The listing builds one solid part. Answer for the finished solid, in the listing's coordinates (mm). A direction names the side the tool comes from. Coordinates: 2 decimals unless noted, no trailing zeros. Write each loop counter-clockwise with the first axis right and the second up, starting at its lowest first coordinate (ties: lowest second). Pieces come first, ordered by that corner, then holes. Notation, with made-up numbers: M 69,-13 L 112,-13 A26 cw 112,16 Z; hole C -23.5,25 d3. An arc over 180 degrees is marked long. Answer as a JSON object with one key per item and string values. Group by question number.
from build123d import *

# Parameters (mm, degrees)
SKETCH1_R           = 6
SKETCH1_R_2         = 2.5
BOSS_EXTRUDE1_DEPTH = 11.75
SKETCH2_R           = 2.413
SKETCH3_R           = 1.5
CUT_EXTRUDE1_DEPTH  = 12
CHAMFER1_SIZE       = 0.508
CHAMFER2_SIZE       = 0.254


with BuildPart() as part:
    # Sketch1 → Boss-Extrude1 (new body)
    with BuildSketch(Plane(origin=(0, 0, 0), x_dir=(0, 0, -1), z_dir=(1, 0, 0))):
        Circle(SKETCH1_R)
        Circle(SKETCH1_R_2, mode=Mode.SUBTRACT)
    extrude(amount=-BOSS_EXTRUDE1_DEPTH)

    # Sketch2 → Cut-Revolve1 (revolve, cut)
    with BuildSketch(Plane(origin=(0, 0, 0), x_dir=(1, 0, 0), z_dir=(0, 1, 0))):
        with Locations((-3.629714112, 7.913)):
            Circle(SKETCH2_R)
    revolve(axis=Axis((0, 0, 0), (1, 0, 0)), mode=Mode.SUBTRACT)

    # Sketch3 → Cut-Extrude1 (cut)
    with BuildSketch(Plane(origin=(0, 0, 0), x_dir=(1, 0, 0), z_dir=(0, 1, 0))):
        with Locations((-8, 0)):
            Circle(SKETCH3_R)
    extrude(amount=CUT_EXTRUDE1_DEPTH, mode=Mode.SUBTRACT)

    # Chamfer1
    chamfer1_edges = [part.edges().sort_by_distance(p)[0] for p in [
        (0, 0, 6),
        (-11.75, 0, 6),
    ]]
    chamfer(chamfer1_edges, length=CHAMFER1_SIZE)

    # Chamfer2
    chamfer2_edges = [part.edges().sort_by_distance(p)[0] for p in [
        (0, 0, 2.5),
    ]]
    chamfer(chamfer2_edges, length=CHAMFER2_SIZE)


solid = part.part
Item 1: Consider L1, parallel to X at y = 3.15, z = 0; L2, parallel to Z at x = -8, y = 4.55; L3, parallel to Y at x = -6.75, z = 0. Determine where each line is inside the solid, lowest interval first. Write a range as from..to.
Item 2: A cutting plane is placed at B-B, the plane z = 0. Write down the section's boundary in (x, y), and give its area (3 significant figures).
Item 3: A tool of negligible diameter and unlimited length cuts with its end or side. For faces 1 (the face through (-11.75, 3, 0)), 2 (the face through (-6.614, 3.974, 0.575)), from which of +Z, -Z, +X, -X, +Y, -Y can it reach the whole face along a straight path? Write none if from no direction.
Item 4: For a pull along Z with two mould halves and no side action, classify faces 3 (the face through (-8.128, -5.857, 1.301)), 4 (the face through (0, 3, -1)), 5 (the face through (-5.92, -2.44, 0.54)) as +Z half, -Z half, draft (parallel to the pull), parting line (faces both ways), or undercut.
Item 5: A cutting plane is placed at D-D, the plane x = -7.25. Write down the section's boundary in (y, z).
Item 6: A cutting plane is placed at A-A, the plane y = 0. Write down the section's boundary in (x, z), and give its area (3 significant figures).
Item 7: Flat-ended cylindrical pins translate along their axes: pin 1 Ø4 at (x, z) = (-1.5, -4) entering from -Y; pin 2 Ø3 at (x, z) = (-8.5, 1.5) entering from +Y; pin 3 Ø1 at (x, y) = (-1.5, -1) entering from +Z. Find the tip coordinate at first contact, or state that the pin passes through.
Item 8: A cutting plane is placed at C-C, the plane x = -3. Write down the section's boundary in (y, z), and give its area (3 significant figures).
Answer:
{
 "1": {"L1": "-11.75..-9.5, -6.5..0", "L2": "-3.91..-1.5, 1.5..3.91", "L3": "-6..-2.5"},
 "2": {"outline": "M -11.75,-5.49 L -11.24,-6 L -5.1,-6 A2.41 cw -2.16,-6 L -0.51,-6 L 0,-5.49 L 0,-2.75 L -0.25,-2.5 L -11.75,-2.5 Z; M -11.75,2.5 L -9.5,2.5 L -9.5,6 L -11.24,6 L -11.75,5.49 Z; M -6.5,2.5 L -0.25,2.5 L 0,2.75 L 0,5.49 L -0.51,6 L -2.16,6 A2.41 cw -5.1,6 L -6.5,6 Z", "area": "69.2 mm2"},
 "3": {"face 1": "+Z, -Z, -X, +Y, -Y", "face 2": "+Y"},
 "4": {"face 3": "parting line", "face 4": "draft", "face 5": "undercut"},
 "5": {"outline": "M 2.14,-1.3 A2.5 cw long 2.14,1.3 L 5.86,1.3 A6 ccw long 5.86,-1.3 Z"},
 "6": {"outline": "M -11.75,-5.49 L -11.24,-6 L -5.1,-6 A2.41 cw -2.16,-6 L -0.51,-6 L 0,-5.49 L 0,-2.75 L -0.25,-2.5 L -11.75,-2.5 Z; M -11.75,2.5 L -0.25,2.5 L 0,2.75 L 0,5.49 L -0.51,6 L -2.16,6 A2.41 cw -5.1,6 L -11.24,6 L -11.75,5.49 Z", "area": "79.7 mm2"},
 "7": {"pin 1": "y = -5.66", "pin 2": "y = 5.99", "pin 3": "z = 5.98"},
 "8": {"outline": "C 0,0 d11.17; hole C 0,0 d5", "area": "78.3 mm2"}
}
